```python
from build123d import *

# Parameters (mm, degrees)
SKETCH1_W           = 80
SKETCH1_H           = 5
SKETCH1_W_2         = 3
SKETCH1_H_2         = 3
BOSS_EXTRUDE1_DEPTH = 5
SKETCH2_W           = 3
SKETCH2_H           = 3
CUT_EXTRUDE1_DEPTH  = 5


with BuildPart() as part:
    # Sketch1 → Boss-Extrude1 (new body)
    with BuildSketch(Plane.XY):
        with Locations((40, 2.5)):
            Rectangle(SKETCH1_W, SKETCH1_H)
        with Locations((54.85, 2.5)):
            Rectangle(SKETCH1_W_2, SKETCH1_H_2, mode=Mode.SUBTRACT)
        with Locations((25, 2.5)):
            Rectangle(SKETCH1_W_2, SKETCH1_H_2, mode=Mode.SUBTRACT)
    extrude(amount=BOSS_EXTRUDE1_DEPTH)

    # Sketch2 → Cut-Extrude1 (cut)
    with BuildSketch(Plane(origin=(0, 5, 0), x_dir=(1, 0, 0), z_dir=(0, 1, 0))):
        with Locations((77.5, -2.5)):
            Rectangle(SKETCH2_W, SKETCH2_H)
        with Locations((2.5, -2.5)):
            Rectangle(SKETCH2_W, SKETCH2_H)
        with Locations((11.5, -2.5)):
            Rectangle(SKETCH2_W, SKETCH2_H)
        with Locations((68.5, -2.5)):
            Rectangle(SKETCH2_W, SKETCH2_H)
    extrude(amount=-CUT_EXTRUDE1_DEPTH, mode=Mode.SUBTRACT)


solid = part.part
```
Model file for the job. Use its own axes, mm. A direction names the side the tool comes from. Round coordinates to 2 decimals unless told otherwise and drop trailing zeros. Write each loop counter-clockwise with the first axis right and the second up, starting at its lowest first coordinate (ties: lowest second). Pieces come first, ordered by that corner, then holes. Notation, with made-up numbers: (-14, 73) -> (-1, 73) arc R31 cw to (-1, 107) -> close; hole circle Ø6 at (43.25, 65.25). An arc over 180 degrees is marked (long way). Answer as CSV lines item,"result".
1. Slice it at A-A, the plane y = 2. List the corners of the cut face in (x, z), plus the area to 3 significant figures.
Resolved:
outline,"(0, 0) -> (23.5, 0) -> (23.5, 5) -> (0, 5) -> close; (26.5, 0) -> (53.35, 0) -> (53.35, 5) -> (26.5, 5) -> close; (56.35, 0) -> (80, 0) -> (80, 5) -> (56.35, 5) -> close; hole (1, 1) -> (4, 1) -> (4, 4) -> (1, 4) -> close; hole (10, 1) -> (13, 1) -> (13, 4) -> (10, 4) -> close; hole (67, 1) -> (70, 1) -> (70, 4) -> (67, 4) -> close; hole (76, 1) -> (79, 1) -> (79, 4) -> (76, 4) -> close"
area,"334 mm²"
2. Drill centre lines: line 1 (X direction, y = 3.6, z = 0.95); line 2 (X direction, y = 4.15, z = 1.9); line 3 (Z direction, x = 68.5, y = 1.4). Where is each one in solid material? Low to high.
Resolved:
line 1,"0 to 23.5, 26.5 to 53.35, 56.35 to 80"
line 2,"0 to 1, 4 to 10, 13 to 67, 70 to 76, 79 to 80"
line 3,"0 to 1, 4 to 5"
3. Mould opens along Y. For faces 4 (the face through (39, 5, 2)), 5 (the face through (70, 3, 3)), 6 (the face through (55, 4, 2)) say: +Y half, -Y half, draft (parallel to the pull), parting line (faces both ways), or undercut.
Resolved:
face 4,"+Y half"
face 5,"draft"
face 6,"undercut"
4. Tool access for faces 1 (the face through (2, 3, 4)), 2 (the face through (56.35, 2, 2)), 3 (the face through (39, 3, 5)): list every direction of +Z, -Z, +X, -X, +Y, -Y with a clear straight run to the whole face (end or side of a thin tool).
Resolved:
face 1,"+Y, -Y"
face 2,"+Z, -Z"
face 3,"+Z, +X, -X, +Y, -Y"
5. Slice it at B-B, the plane z = 2.2. List the corners of the cut face in (x, y), plus the area to 3 significant figures.
Resolved:
outline,"(0, 0) -> (1, 0) -> (1, 5) -> (0, 5) -> close; (4, 0) -> (10, 0) -> (10, 5) -> (4, 5) -> close; (13, 0) -> (67, 0) -> (67, 5) -> (13, 5) -> close; (70, 0) -> (76, 0) -> (76, 5) -> (70, 5) -> close; (79, 0) -> (80, 0) -> (80, 5) -> (79, 5) -> close; hole (23.5, 1) -> (26.5, 1) -> (26.5, 4) -> (23.5, 4) -> close; hole (53.35, 1) -> (56.35, 1) -> (56.35, 4) -> (53.35, 4) -> close"
area,"322 mm²"
